For this review, use the dimensioned drawing (mm, ordinates from the lowest corner) and the shaded views. Round coordinates to 2 decimals unless told otherwise and drop trailing zeros. Order: outer loops, then holes, each group sorted by start corner. A loop starts at its lowest first (then second) coordinate and runs counter-clockwise, first axis right, second up. Notation, with made-up numbers: (-9, -30.75) - (14, -30.75) arc R29 cw to (14, 6.25) - close; hole circle Ø7 at (21.25, -20). An arc over 180 degrees is marked (long way). Write item = value, one per line.
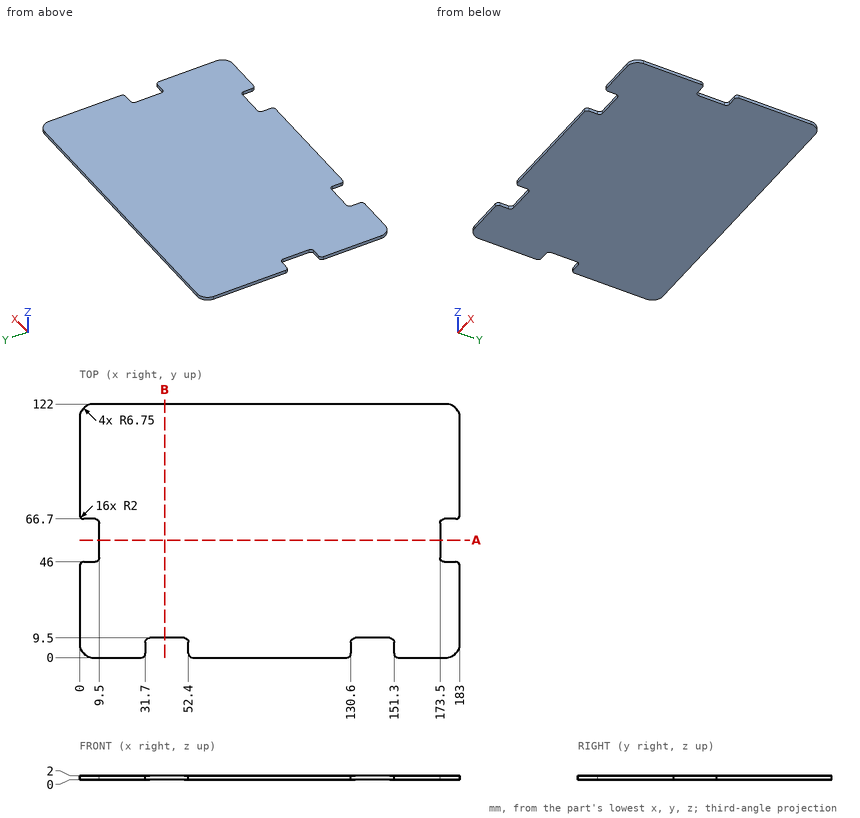
1) To check wall thickness, follow L1, parallel to Y at x = 139.5, z = 1.85; L2, parallel to X at y = 55.5, z = 0.3; L3, parallel to Y at x = 33, z = 1.6. State the ranges of each line that lie inside material, in increasing order. Write a range as from..to.
Findings:
L1 = 9.5..122
L2 = 9.5..173.5
L3 = 9.37..122
2) We need section A-A on y = 56.5. Write out the cut boundary in (x, z), and give its area (3 significant figures).
Findings:
outline = (9.5, 0) - (173.5, 0) - (173.5, 2) - (9.5, 2) - close
area = 328 mm^2
3) We need section B-B on x = 41. Write out the cut boundary in (y, z), and give its area (3 significant figures).
Findings:
outline = (9.5, 0) - (122, 0) - (122, 2) - (9.5, 2) - close
area = 225 mm^2
4) Clearance check with flat-ended pins moving along their axes: pin 1 Ø0.6 at (y, z) = (4.5, 1) entering from -X; pin 2 Ø1 at (x, z) = (130, 1) entering from -Y; pin 3 Ø0.6 at (y, z) = (53, 1) entering from -X. State where each tip first meets the part, or that it passes through.
Findings:
pin_1 = 0.29
pin_2 = 0.21
pin_3 = 9.5
